```python
from build123d import *

# Parameters (mm, degrees)
SKETCH1_R           = 6
SKETCH1_R_2         = 1.7
SKETCH1_R_3         = 1
SKETCH1_R_4         = 0.6
BASEPLATE_DEPTH     = 1
SKETCH1_3_R         = 0.6
SCREWHOLES_DEPTH    = 2
SKETCH1_4_R         = 1
SKETCH1_4_R_2       = 0.6
SCREWHATSLOTS_DEPTH = 0.5
SKETCH2_R           = 2
BEARINGSLOT_DEPTH   = 0.5


with BuildPart() as part:
    # Sketch1 → BasePlate (new body)
    with BuildSketch(Plane(origin=(0, 0, 0), x_dir=(1, 0, 0), z_dir=(0, 1, 0))):
        Circle(SKETCH1_R)
        Circle(SKETCH1_R_2, mode=Mode.SUBTRACT)
        with Locations((0, 4)):
            Circle(SKETCH1_R_3, mode=Mode.SUBTRACT)
        with Locations((0, -4)):
            Circle(SKETCH1_R_3, mode=Mode.SUBTRACT)
        with Locations((0, -4)):
            Circle(SKETCH1_R_4)
        with Locations((0, 4)):
            Circle(SKETCH1_R_4)
        with Locations((0, 4)):
            Circle(SKETCH1_R_3)
        with Locations((0, 4)):
            Circle(SKETCH1_R_4, mode=Mode.SUBTRACT)
        with Locations((0, -4)):
            Circle(SKETCH1_R_3)
        with Locations((0, -4)):
            Circle(SKETCH1_R_4, mode=Mode.SUBTRACT)
    extrude(amount=BASEPLATE_DEPTH)

    # Sketch1<3> → ScrewHoles (cut, through all)
    with BuildSketch(Plane(origin=(0, 0, 0), x_dir=(1, 0, 0), z_dir=(0, 1, 0))):
        with Locations((0, -4)):
            Circle(SKETCH1_3_R)
        with Locations((0, 4)):
            Circle(SKETCH1_3_R)
    extrude(amount=SCREWHOLES_DEPTH, mode=Mode.SUBTRACT)

    # Sketch1<4> → ScrewHatSlots (cut)
    with BuildSketch(Plane(origin=(0, 0, 0), x_dir=(1, 0, 0), z_dir=(0, 1, 0))):
        with Locations((0, -4)):
            Circle(SKETCH1_4_R)
        with Locations((0, -4)):
            Circle(SKETCH1_4_R_2, mode=Mode.SUBTRACT)
        with Locations((0, 4)):
            Circle(SKETCH1_4_R)
        with Locations((0, 4)):
            Circle(SKETCH1_4_R_2, mode=Mode.SUBTRACT)
    extrude(amount=SCREWHATSLOTS_DEPTH, mode=Mode.SUBTRACT)

    # Sketch2 → BearingSlot (cut)
    with BuildSketch(Plane(origin=(0, 1, 0), x_dir=(1, 0, 0), z_dir=(0, 1, 0))):
        Circle(SKETCH2_R)
    extrude(amount=-BEARINGSLOT_DEPTH, mode=Mode.SUBTRACT)


solid = part.part
```
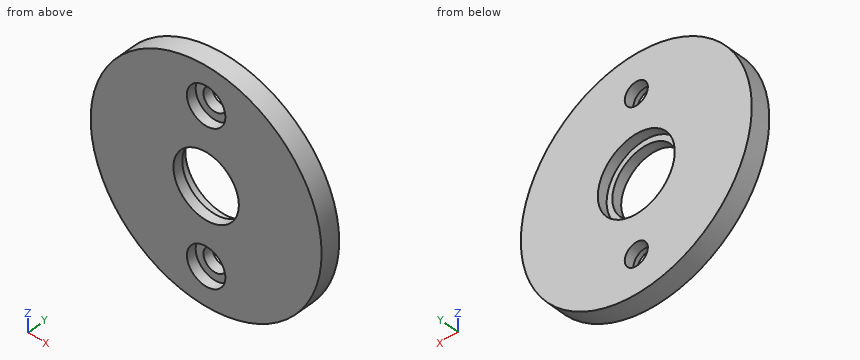
Geometry: final body of the model. Coordinates: model frame, mm. Round coordinates to 2 decimals unless told otherwise and drop trailing zeros. Order: outer loops, then holes, each group sorted by start corner. A loop starts at its lowest first (then second) coordinate and runs counter-clockwise, first axis right, second up. Notation, with made-up numbers: M 57,-26 L 61,-26 A12 cw 61,-16 Z; hole C -26.75,86.5 d3. An arc over 180 degrees is marked long. One line per item, written item: value.
(1) Line query: probe 1 along Z at (x, y) = (0, 0.7); probe 2 along Z at (x, y) = (0, 0.3); probe 3 along X at (y, z) = (0.75, 0). Output: solid intervals per line, ascending. Write a range as [from, to].
Result sheet:
probe 1: [-6, -4.6], [-3.4, -2], [2, 3.4], [4.6, 6]
probe 2: [-6, -5], [-3, -1.7], [1.7, 3], [5, 6]
probe 3: [-6, -2], [2, 6]
(2) Cut plane B-B (y = 0.8). Return the cut outline in (x, z), and give its area (3 significant figures).
Result sheet:
outline: C 0,0 d12; hole C 0,0 d4; hole C 0,-4 d1.2; hole C 0,4 d1.2
area: 98.3 mm2
(3) Cut plane D-D (x = 5). Return the cut outline in (y, z), and give its area (3 significant figures).
Result sheet:
outline: M 0,-3.32 L 1,-3.32 L 1,3.32 L 0,3.32 Z
area: 6.63 mm2
(4) Cut plane A-A (z = 0). Return the cut outline in (x, y).
Result sheet:
outline: M -6,0 L -1.7,0 L -1.7,0.5 L -2,0.5 L -2,1 L -6,1 Z; M 1.7,0 L 6,0 L 6,1 L 2,1 L 2,0.5 L 1.7,0.5 Z
(5) Pin query (flat end, axial travel): P1, Ø5, axis at x = 2, z = -1.5, coming from the -Y side; P2, Ø1.9, axis at x = 0, z = -4, coming from the -Y side; P3, Ø1.1, axis at x = 0, z = 4, coming from the -Y side. Return the tip coordinate at first contact, or that it passes through.
Result sheet:
P1: y = 0
P2: y = 0.5
P3: through
(6) Cut plane C-C (z = 4). Return the cut outline in (x, y).
Result sheet:
outline: M -4.47,0 L -1,0 L -1,0.5 L -0.6,0.5 L -0.6,1 L -4.47,1 Z; M 0.6,0.5 L 1,0.5 L 1,0 L 4.47,0 L 4.47,1 L 0.6,1 Z
